```python
from build123d import *

# Parameters (mm, degrees)
F1_DEPTH     = 25.4
F2_DEPTH     = 12.7
F3_T4_DEPTH  = 139.4853841596
F3_S5_R      = 56.9586140596
F3_T6_DEPTH  = 72
F3_T11_DEPTH = 84.4927710193
F3_S12_R     = 29.500157879
F3_T13_DEPTH = 46
F3_T15_ANGLE = 154.3366921311


# Not quite as in the source:
# - a fillet or chamfer that OpenCascade refuses, or shapes differently, is made with other operations: its cross-section is extruded or revolved along the edge and cut away or added


with BuildPart() as f1:
    # F0 (on Top) → F1 (new body)
    with BuildSketch(Plane.XY):
        with BuildLine():
            ThreePointArc((-44.6654795557, 14.8543386834), (-41.6735799491, 7.6933988578), (-40.6527291, 0))
            Line((-40.6527291, 0), (-2.5527291, 0))
            Line((-2.5527291, 0), (-2.5527291, 130.3065121174))
            Line((-2.5527291, 130.3065121174), (-70.1528869789, 130.3065121174))
            Line((-70.1528869789, 130.3065121174), (-70.1528869789, 48.7239612584))
            ThreePointArc((-70.1528869789, 48.7239612584), (-54.141159867, 34.2483874097), (-44.6654795557, 14.8543386834))
        make_face()
    extrude(amount=F1_DEPTH)

    # F0 (on Top) → F2 (join)
    with BuildSketch(Plane.XY):
        with BuildLine():
            Line((-42.6944307983, 0), (-70.1528869789, 0))
            Line((-70.1528869789, 0), (-70.1528869789, 29.500157879))
            ThreePointArc((-70.1528869789, 29.500157879), (-95.730852606, -14.6978566215), (-44.6654795557, -14.8543386834))
            ThreePointArc((-44.6654795557, -14.8543386834), (-43.1893431296, -7.4922695314), (-42.6944307983, 0))
        make_face()
        with BuildLine():
            ThreePointArc((-44.6654795557, 14.8543386834), (-43.1893431296, 7.4922695314), (-42.6944307983, 0))
            Line((-42.6944307983, 0), (-40.6527291, 0))
            ThreePointArc((-40.6527291, 0), (-41.6735799491, 7.6933988578), (-44.6654795557, 14.8543386834))
        make_face()
        with BuildLine():
            Line((-40.6527291, 0), (-42.6944307983, 0))
            ThreePointArc((-42.6944307983, 0), (-43.1893431296, -7.4922695314), (-44.6654795557, -14.8543386834))
            ThreePointArc((-44.6654795557, -14.8543386834), (-41.6735799491, -7.6933988578), (-40.6527291, 0))
        make_face()
        with BuildLine():
            ThreePointArc((-44.6654795557, -14.8543386834), (-95.730852606, -14.6978566215), (-70.1528869789, 29.500157879))
            Line((-70.1528869789, 29.500157879), (-70.1528869789, 48.7239612584))
            ThreePointArc((-70.1528869789, 48.7239612584), (-152.5216924476, -21.1940986511), (-44.6654795557, -14.8543386834))
        make_face()
        with BuildLine():
            Line((-70.1528869789, 48.7239612584), (-70.1528869789, 29.500157879))
            ThreePointArc((-70.1528869789, 29.500157879), (-55.4550303574, 25.577965627), (-44.6654795557, 14.8543386834))
            ThreePointArc((-44.6654795557, 14.8543386834), (-54.141159867, 34.2483874097), (-70.1528869789, 48.7239612584))
        make_face()
        with BuildLine():
            ThreePointArc((-44.6654795557, 14.8543386834), (-41.6735799491, 7.6933988578), (-40.6527291, 0))
            Line((-40.6527291, 0), (-2.5527291, 0))
            Line((-2.5527291, 0), (-2.5527291, 130.3065121174))
            Line((-2.5527291, 130.3065121174), (-70.1528869789, 130.3065121174))
            Line((-70.1528869789, 130.3065121174), (-70.1528869789, 48.7239612584))
            ThreePointArc((-70.1528869789, 48.7239612584), (-54.141159867, 34.2483874097), (-44.6654795557, 14.8543386834))
        make_face()
    extrude(amount=F2_DEPTH)

    # F3: fillet of radius 25.4 on 2 edges, made by hand


with BuildPart() as f3_tool2:
    # F3_s3 → F3_t4 (new body)
    with BuildSketch(Plane.XZ.offset(54.9926131403)):
        with BuildLine():
            ThreePointArc((-92.1499322351, 12.7), (-79.4499322351, 9.2970452561), (-70.1528869789, 0))
            Line((-70.1528869789, 0), (-69.7129460738, 0.254))
            ThreePointArc((-69.7129460738, 0.254), (-69.6448869789, 6.35), (-69.6448869789, 12.7))
            Line((-69.6448869789, 12.7), (-70.1528869789, 13.208))
            Line((-70.1528869789, 13.208), (-92.1499322351, 13.208))
            Line((-92.1499322351, 13.208), (-92.1499322351, 12.7))
        make_face()
    extrude(amount=-F3_T4_DEPTH)

    # F3_s5 → F3_t6 (cut, symmetric)
    with BuildSketch(Plane.XY.offset(6.6)):
        with Locations((-99.6530448579, 0)):
            Circle(F3_S5_R)
    extrude(amount=F3_T6_DEPTH, both=True, mode=Mode.SUBTRACT)

    split(bisect_by=Plane.XZ, keep=Keep.TOP)


with BuildPart() as f1_1:
    add(f1.part)

    # F3_t1: cut F3_tool2
    add(f3_tool2.part, mode=Mode.SUBTRACT)


with BuildPart() as f3_tool9:
    # F3_s10 → F3_t11 (new body)
    with BuildSketch(Plane.XZ):
        with BuildLine():
            ThreePointArc((-92.1499322351, 12.7), (-79.4499322351, 9.2970452561), (-70.1528869789, 0))
            Line((-70.1528869789, 0), (-69.7129460738, 0.254))
            ThreePointArc((-69.7129460738, 0.254), (-69.6448869789, 6.35), (-69.6448869789, 12.7))
            Line((-69.6448869789, 12.7), (-70.1528869789, 13.208))
            Line((-70.1528869789, 13.208), (-92.1499322351, 13.208))
            Line((-92.1499322351, 13.208), (-92.1499322351, 12.7))
        make_face()
    extrude(amount=-F3_T11_DEPTH)

    # F3_s12 → F3_t13 (intersect, symmetric)
    with BuildSketch(Plane.XY.offset(6.6)):
        with Locations((-70.1528869789, 0)):
            Circle(F3_S12_R)
    extrude(amount=F3_T13_DEPTH, both=True, mode=Mode.INTERSECT)


with BuildPart() as f1_2:
    add(f1_1.part)

    # F3_t8: cut F3_tool9
    add(f3_tool9.part, mode=Mode.SUBTRACT)

    # F3_s14 → F3_t15 (revolve, cut)
    with BuildSketch(Plane(origin=(-82.9981282802, -37.1796571073, 0), x_dir=(0, 0, 1), z_dir=(-0.912617648, -0.4088141736, 0))):
        with BuildLine():
            ThreePointArc((25.4, 119.695236496), (21.9970452561, 106.995236496), (12.7, 97.6981912399))
            Line((12.7, 97.6981912399), (12.954, 97.2582503348))
            ThreePointArc((12.954, 97.2582503348), (19.05, 97.1901912399), (25.4, 97.1901912399))
            Line((25.4, 97.1901912399), (25.908, 97.6981912399))
            Line((25.908, 97.6981912399), (25.908, 119.695236496))
            Line((25.908, 119.695236496), (25.4, 119.695236496))
        make_face()
    revolve(axis=Axis((-99.6530448579, 0, 25.4), (0, 0, -1)), revolution_arc=F3_T15_ANGLE, mode=Mode.SUBTRACT)


solid = f1_2.part
```
The listing builds one solid part. Answer for the finished solid, in the listing's coordinates (mm). A direction names the side the tool comes from. Give positions to 0.01 mm unless a question says otherwise; leave off trailing zeros. Order: outer loops, then holes, each group sorted by start corner. A loop starts at its lowest first (then second) coordinate and runs counter-clockwise, first axis right, second up. Notation, with made-up numbers: (-22.75, 69.25) -> (-17.75, 69.25) arc R27 cw to (-17.75, 101.25) -> close; hole circle Ø3 at (59, -16). An arc over 180 degrees is marked (long way). Answer as CSV lines item,"result". Start each with the question number.
Q1. A cutting plane is placed at A-A (z = 4). Determine the outline of the cut face in (x, y), then the cut area to 3 significant figures.
Q2. Which of the six approach directions +Z, -Z, +X, -X, +Y, -Y give full straight-line access (tool end or side, diameter ignored) to faces 1 (the flat face through (-29, 81, 25.4)), 2 (the flat face through (-22, 0, 13)), 3 (the flat face through (-62, 0, 6)), 4 (the cylindrical face through (-43.203, 7.597, 6.261)), 5 (the cylindrical face through (-41.294, 6.118, 13.851))?
Q3. A cutting plane is placed at C-C (z = 17.75). Determine the outline of the cut face in (x, y).
Q4. A cutting plane is placed at B-B (y = 89). Determine the outline of the cut face in (x, z).
Q5. Given pin 1 (7.5 mm diameter, centred on y = 99.5, z = 7.5, fed in from -X); pin 2 (6 mm diameter, centred on y = 41.5, z = 16, fed in from -X); pin 3 (5 mm diameter, centred on x = -95.5, z = 9, fed in from +Y), each flat-ended and moving along its own axis, determine where each tip first touches the part or whether it passes through.
Q6. A cutting plane is placed at D-D (x = -141.5). Determine the outline of the cut face in (y, z).
Q7. Find the intervals of material crossed by L1, parallel to Y at x = -26.5, z = 14.5; L2, parallel to X at y = 122, z = 22.5; L3, parallel to Z at x = -122, y = 43, in increasing order.
Results found:
1,outline,"(-70.15, 48.72) arc R56.96 ccw (long way) to (-44.67, -14.85) arc R29.5 ccw to (-40.65, 0) -> (-2.55, 0) -> (-2.55, 130.31) -> (-70.15, 130.31) -> close; hole (-73.01, 0) -> (-42.69, 0) arc R56.96 ccw to (-44.67, 14.85) arc R29.5 ccw to (-73.01, 29.36) -> close"
1,area,"17,300 mm2"
2,face 1,"+Z, +X, -X, +Y, -Y"
2,face 2,"+Z, -Z, +X, -Y"
2,face 3,"+Z"
2,face 4,"+Z, -Z"
2,face 5,"+Z, -X, -Y"
3,outline,"(-70.15, 53.15) arc R60.79 cw to (-38.87, 0) -> (-2.55, 0) -> (-2.55, 130.31) -> (-70.15, 130.31) -> close"
4,outline,"(-70.15, 0) -> (-2.55, 0) -> (-2.55, 25.4) -> (-70.15, 25.4) -> close"
5,pin 1,"x = -70.15"
5,pin 2,"x = -61.92"
5,pin 3,"y = 56.93"
6,outline,"(-38.64, 0) -> (38.64, 0) -> (38.64, 12.7) -> (-38.64, 12.7) -> close"
7,L1,"0 to 130.31"
7,L2,"-70.15 to -2.55"
7,L3,"0 to 12.7"
